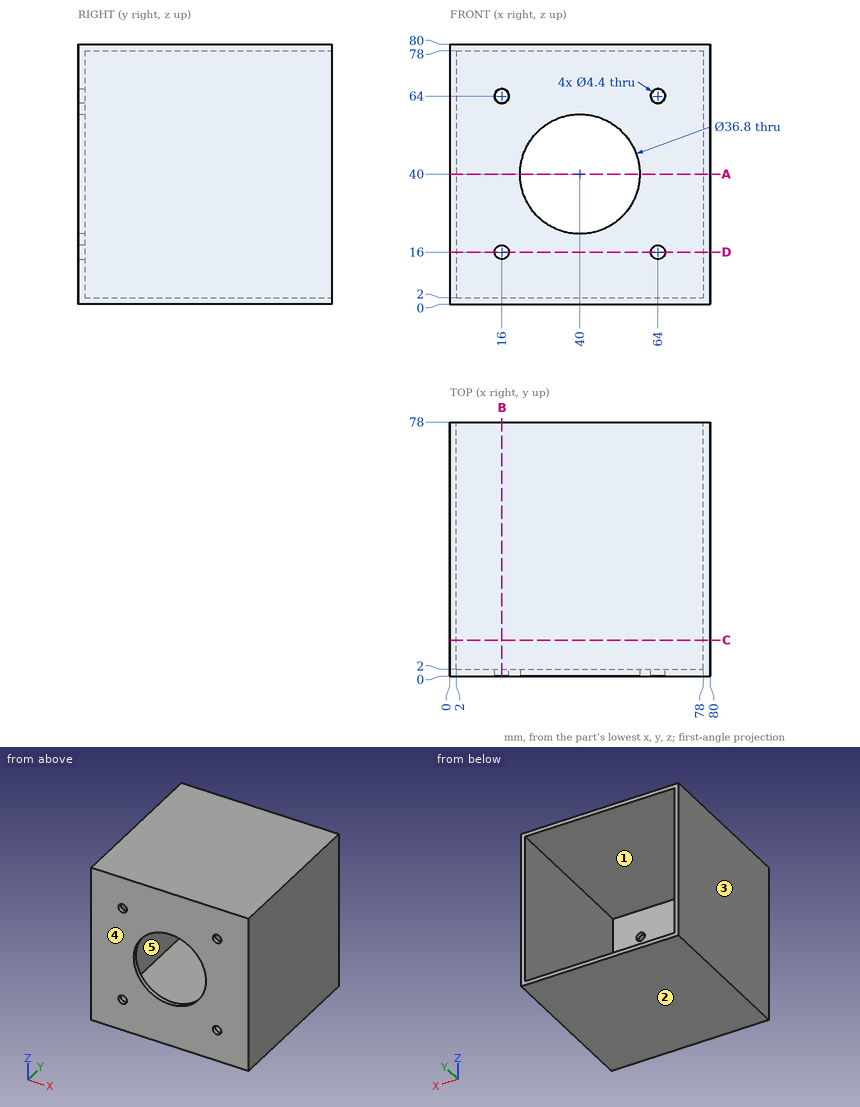
The figure shows three views and two pictorial views of one solid part (mm, origin at its lowest corner). Answer the questions. A direction names the side the tool comes from. Give positions to 0.01 mm unless a question says otherwise; leave off trailing zeros. Order: outer loops, then holes, each group sorted by start corner. A loop starts at its lowest first (then second) coordinate and runs counter-clockwise, first axis right, second up. Notation, with made-up numbers: (85.5, 31) -> (144.5, 31) arc R36 cw to (144.5, 65) -> close; hole circle Ø10 at (19.5, -19.5). An arc over 180 degrees is marked (long way). Answer as CSV lines item,"result". Start each with the question number.
Q1. Determine the mould class of the marked faces 1, 2 and 3 for opening direction Z: pulls with the +Z half, pulls with the -Z half, needs draft (parallel to the pull), parting line crosses it, or undercut.
Q2. A cutting plane is placed at D-D (z = 16). Determine the outline of the cut face in (x, y).
Q3. Which of the six approach directions +Z, -Z, +X, -X, +Y, -Y give full straight-line access (tool end or side, diameter ignored) to the marked faces 4 and 5?
Q4. A cutting plane is placed at A-A (z = 40). Determine the outline of the cut face in (x, y).
Q5. A cutting plane is placed at C-C (y = 11). Determine the outline of the cut face in (x, z).
Q6. A cutting plane is placed at B-B (x = 16). Determine the outline of the cut face in (y, z), then the cut area to 3 significant figures.
Q7. Given pin 1 (8 mm diameter, centred on x = 56.5, z = 51, fed in from +Y); pin 2 (2.5 mm diameter, centred on x = 64, z = 16, fed in from +Y), each flat-ended and moving along its own axis, determine where each tip first touches the part or whether it passes through.
Q8. Find the intervals of material crossed by L1, parallel to X at y = 1, z = 64; L2, parallel to X at y = 46, z = 25, in increasing order.
Results found:
1,face 1,"undercut"
1,face 2,"pulls with the -Z half"
1,face 3,"needs draft"
2,outline,"(0, 0) -> (13.8, 0) -> (13.8, 2) -> (2, 2) -> (2, 78) -> (0, 78) -> close; (18.2, 0) -> (61.8, 0) -> (61.8, 2) -> (18.2, 2) -> close; (66.2, 0) -> (80, 0) -> (80, 78) -> (78, 78) -> (78, 2) -> (66.2, 2) -> close"
3,face 4,"+Z, -Z, +X, -X, -Y"
3,face 5,"+Y"
4,outline,"(0, 0) -> (21.6, 0) -> (21.6, 2) -> (2, 2) -> (2, 78) -> (0, 78) -> close; (58.4, 0) -> (80, 0) -> (80, 78) -> (78, 78) -> (78, 2) -> (58.4, 2) -> close"
5,outline,"(0, 0) -> (80, 0) -> (80, 80) -> (0, 80) -> close; hole (2, 2) -> (78, 2) -> (78, 78) -> (2, 78) -> close"
6,outline,"(0, 0) -> (78, 0) -> (78, 2) -> (2, 2) -> (2, 13.8) -> (0, 13.8) -> close; (0, 18.2) -> (2, 18.2) -> (2, 61.8) -> (0, 61.8) -> close; (0, 66.2) -> (2, 66.2) -> (2, 78) -> (78, 78) -> (78, 80) -> (0, 80) -> close"
6,area,"446 mm2"
7,pin 1,"y = 2"
7,pin 2,"through"
8,L1,"0 to 13.8, 18.2 to 61.8, 66.2 to 80"
8,L2,"0 to 2, 78 to 80"
